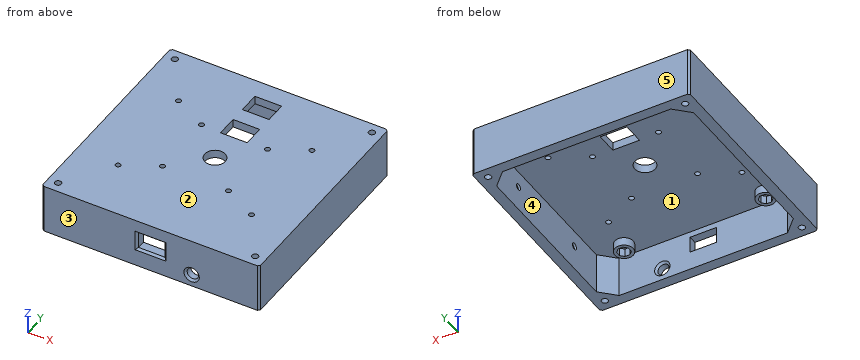
from build123d import *

# Parameters (mm, degrees)
SKETCH1_W               = 106
SKETCH1_H               = 106
BOSS_EXTRUDE1_DEPTH     = 4
SKETCH2_W               = 106
SKETCH2_H               = 106
BOSS_EXTRUDE2_DEPTH     = 20
SKETCH7_R               = 1.55
CUT_EXTRUDE2_DEPTH      = 50
SKETCH8_R               = 1.25
SKETCH8_R_2             = 5
SKETCH8_W               = 13
SKETCH8_H               = 10.3
CUT_EXTRUDE3_DEPTH      = 10
SKETCH9_R               = 4.5
BOSS_EXTRUDE3_DEPTH     = 4
SKETCH14_R              = 2.75
SKETCH14_W              = 13
SKETCH14_H              = 8
CUT_EXTRUDE4_DEPTH      = 10
CHAMFER1_SIZE           = 1
CHAMFER2_SIZE           = 1
CUT_EXTRUDE5_DEPTH      = 97
CUT_EXTRUDE5_DEPTH_BACK = 1
SKETCH15_R              = 1.6
CHAMFER3_SIZE           = 1


with BuildPart() as part:
    # Sketch1 → Boss-Extrude1 (new body)
    with BuildSketch(Plane.XY):
        Rectangle(SKETCH1_W, SKETCH1_H)
    extrude(amount=-BOSS_EXTRUDE1_DEPTH)

    # Sketch2 → Boss-Extrude2 (add)
    with BuildSketch(Plane(origin=(0, 0, -4), x_dir=(-1, 0, 0), z_dir=(0, 0, -1))):
        Rectangle(SKETCH2_W, SKETCH2_H)
        Polygon((-48, 41), (-48, -41), (-41, -48), (41, -48), (48, -41), (48, 41), (41, 48), (-41, 48), align=None, mode=Mode.SUBTRACT)
    extrude(amount=BOSS_EXTRUDE2_DEPTH)

    # Sketch7 → Cut-Extrude2 (cut)
    with BuildSketch(Plane.XY):
        with Locations((-48, 48)):
            Circle(SKETCH7_R)
        with Locations((48, 48)):
            Circle(SKETCH7_R)
        with Locations((-48, -48)):
            Circle(SKETCH7_R)
        with Locations((48, -48)):
            Circle(SKETCH7_R)
    extrude(amount=-CUT_EXTRUDE2_DEPTH, mode=Mode.SUBTRACT)

    # Sketch8 → Cut-Extrude3 (cut)
    with BuildSketch(Plane.XY):
        with Locations((32.5, 24.9)):
            Circle(SKETCH8_R)
        with Locations((-32.5, 24.9)):
            Circle(SKETCH8_R)
        with Locations((-32.5, -24.9)):
            Circle(SKETCH8_R)
        with Locations((32.5, -24.9)):
            Circle(SKETCH8_R)
        with Locations((16.086679272, -16.086679272)):
            Circle(SKETCH8_R)
        with Locations((-16.086679272, -16.086679272)):
            Circle(SKETCH8_R)
        with Locations((16.086679272, 16.086679272)):
            Circle(SKETCH8_R)
        with Locations((-16.086679272, 16.086679272)):
            Circle(SKETCH8_R)
        Circle(SKETCH8_R_2)
        with Locations((0, 38.65)):
            Rectangle(SKETCH8_W, SKETCH8_H)
        with Locations((0, 20.65)):
            Rectangle(SKETCH8_W, SKETCH8_H)
    extrude(amount=-CUT_EXTRUDE3_DEPTH, mode=Mode.SUBTRACT)

    # Sketch9 → Boss-Extrude3 (add)
    # profile 1 of 4: a face of its own
    with BuildSketch(Plane.XY.offset(-4)):
        with Locations((-34.5, 41)):
            Circle(SKETCH9_R)
        Polygon((-35.701219331, 38.1), (-33.298780669, 38.1), (-31.6, 39.798780669), (-31.6, 42.201219331), (-33.298780669, 43.9), (-35.701219331, 43.9), (-37.4, 42.201219331), (-37.4, 39.798780669), align=None, mode=Mode.SUBTRACT)
    # profile 2 of 4: a face of its own
    with BuildSketch(Plane.XY.offset(-4)):
        with Locations(Location((34.5, 41, 0), (0, 0, 180))):
            Circle(SKETCH9_R)
        Polygon((37.4, 39.798780669), (35.701219331, 38.1), (33.298780669, 38.1), (31.6, 39.798780669), (31.6, 42.201219331), (33.298780669, 43.9), (35.701219331, 43.9), (37.4, 42.201219331), align=None, mode=Mode.SUBTRACT)
    # profile 3 of 4: a face of its own
    with BuildSketch(Plane.XY.offset(-4)):
        with Locations((34.5, -41)):
            Circle(SKETCH9_R)
        Polygon((35.701219331, -38.1), (33.298780669, -38.1), (31.6, -39.798780669), (31.6, -42.201219331), (33.298780669, -43.9), (35.701219331, -43.9), (37.4, -42.201219331), (37.4, -39.798780669), align=None, mode=Mode.SUBTRACT)
    # profile 4 of 4: a face of its own
    with BuildSketch(Plane.XY.offset(-4)):
        with Locations(Location((-34.5, -41, 0), (0, 0, 180))):
            Circle(SKETCH9_R)
        Polygon((-37.4, -39.798780669), (-35.701219331, -38.1), (-33.298780669, -38.1), (-31.6, -39.798780669), (-31.6, -42.201219331), (-33.298780669, -43.9), (-35.701219331, -43.9), (-37.4, -42.201219331), align=None, mode=Mode.SUBTRACT)
    extrude(amount=-BOSS_EXTRUDE3_DEPTH)

    # Sketch14 → Cut-Extrude4 (cut)
    with BuildSketch(Plane.XZ.offset(53)):
        with Locations((20, -18)):
            Circle(SKETCH14_R)
        with Locations((0, -10.83)):
            Rectangle(SKETCH14_W, SKETCH14_H)
    extrude(amount=-CUT_EXTRUDE4_DEPTH, mode=Mode.SUBTRACT)

    # Chamfer1
    chamfer1_edges = [part.edges().sort_by_distance(p)[0] for p in [
        (-53, 53, -12),
        (53, 53, -12),
        (53, -53, -12),
        (-53, -53, -12),
    ]]
    chamfer(chamfer1_edges, length=CHAMFER1_SIZE)

    # Chamfer2
    chamfer2_edges = [part.edges().sort_by_distance(p)[0] for p in [
        (-6.5, -53, -10.83),
        (0, -53, -14.83),
        (6.5, -53, -10.83),
        (0, -53, -6.83),
    ]]
    chamfer(chamfer2_edges, length=CHAMFER2_SIZE)

    # Sketch15 → Cut-Extrude5 (cut, two sides: drawn at the far end of the back side and taken through both)
    with BuildSketch(Plane.ZY.offset(-48).offset(-CUT_EXTRUDE5_DEPTH_BACK)):
        with Locations(Location((-12, -23, 0), (0, 0, 90))):
            Circle(SKETCH15_R)
        with Locations(Location((-12, 23, 0), (0, 0, 90))):
            Circle(SKETCH15_R)
    extrude(amount=CUT_EXTRUDE5_DEPTH + CUT_EXTRUDE5_DEPTH_BACK, mode=Mode.SUBTRACT)

    # Chamfer3
    chamfer3_edges = [part.edges().sort_by_distance(p)[0] for p in [
        (17.25, -48, -18),
        (17.25, -53, -18),
    ]]
    chamfer(chamfer3_edges, length=CHAMFER3_SIZE)


solid = part.part
Model file for the job. Use its own axes, mm. Face numbers are marked on the shaded views. A direction names the side the tool comes from. Round coordinates to 2 decimals unless told otherwise and drop trailing zeros. Order: outer loops, then holes, each group sorted by start corner. A loop starts at its lowest first (then second) coordinate and runs counter-clockwise, first axis right, second up.
(1) Pin check, flat tips, straight feed: pin 1 (12 mm diameter, centred on x = 27, y = -28, fed in from -Z); pin 2 (10 mm diameter, centred on x = 35.5, y = 41, fed in from -Z); pin 3 (2 mm diameter, centred on x = 0.5, y = -50, fed in from +Z). Stop position of each tip, or through.
(2) Pull direction Y, two halves, no side cores. Call the marked faces 1, 2 and 3: released by +Y, released by -Y, zero draft, split by the parting line, or undercut.
(3) 3-axis set-ups, long thin cutter, end or side, ignore diameter. For the marked faces 4 and 5: which of +Z, -Z, +X, -X, +Y, -Y reach the whole face in a straight line?
(4) Band-saw the part on A-A (y = 11.5). List the corners of the cut face in (x, z).
(5) Drill centre lines: line 1 (Y direction, x = 0, z = -1.35); line 2 (Y direction, x = 32.5, z = -1.35); line 3 (X direction, y = -16.5, z = -4.25). Where is each one in solid material? Low to high.
Verdict:
1. pin 1: stops at z = -4
1. pin 2: stops at z = -8
1. pin 3: stops at z = 0
2. face 1: undercut
2. face 2: zero draft
2. face 3: released by -Y
3. face 4: -Z
3. face 5: +Z, -Z, +X, -X, +Y
4. outline: (-53, -24) - (-48, -24) - (-48, -4) - (48, -4) - (48, -24) - (53, -24) - (53, 0) - (-53, 0) - close
5. line 1: y = -53 to -5, 5 to 15.5, 25.8 to 33.5, 43.8 to 53
5. line 2: y = -53 to -26.15, -23.65 to 23.65, 26.15 to 53
5. line 3: x = -53 to -48, 48 to 53
